```python
from build123d import *

# Parameters (mm, degrees)
F1_DEPTH = 120
F3_R     = 2
F4_R     = 3
F5_R     = 1.5


with BuildPart() as f1:
    # F0 (on Right) → F1 (new body)
    with BuildSketch(Plane.YZ):
        Polygon((-10, 19.4), (-10, 0), (0, 0), (0, 4), (-5.7, 4), (-5.7, 16.4), (-3.5, 16.4), (-3.5, 19.4), align=None)
    extrude(amount=F1_DEPTH)

    # F2: F1 across plane


with BuildPart() as f1_1:
    add(f1.part)
    add(f1.part.mirror(Plane.XZ))

    # F3
    f3_edges = [f1_1.edges().sort_by_distance(p)[0] for p in [
        (60, -5.7, 16.4),
        (60, -5.7, 4),
        (60, 5.7, 4),
        (60, 5.7, 16.4),
    ]]
    fillet(f3_edges, radius=F3_R)

    # F4
    f4_edges = [f1_1.edges().sort_by_distance(p)[0] for p in [
        (60, -10, 19.4),
        (60, 10, 19.4),
    ]]
    fillet(f4_edges, radius=F4_R)

    # F5
    f5_edges = [f1_1.edges().sort_by_distance(p)[0] for p in [
        (60, -3.5, 16.4),
        (60, 3.5, 16.4),
    ]]
    fillet(f5_edges, radius=F5_R)


solid = f1_1.part
```
Design review of the part built by this model. Coordinates are the model's own, in mm. A direction names the side the tool comes from. Coordinates: 2 decimals unless noted, no trailing zeros. Order: outer loops, then holes, each group sorted by start corner. A loop starts at its lowest first (then second) coordinate and runs counter-clockwise, first axis right, second up. Notation, with made-up numbers: (-24, 54.25) - (-9, 54.25) arc R27 cw to (-9, 92.25) - close; hole circle Ø9 at (-3, 29). An arc over 180 degrees is marked (long way). Answer in a Markdown table with one row per item.
(1) For faces 4 (the flat face through (59, 5.7, 10)), 5 (the flat face through (0, 0, 3)), list the 3-axis set-ups (+Z, -Z, +X, -X, +Y, -Y) from which the entire face can be reached by the end or side of a thin tool; tool diameter is ignored.
Checked values:
| item | result |
|---|---|
| face 4 | +X, -X |
| face 5 | +Z, -Z, -X, +Y, -Y |
(2) Consider section A-A on z = 7.5. State the section outline as (x, y) points.
Checked values:
| item | result |
|---|---|
| outline | (0, -10) - (120, -10) - (120, -5.7) - (0, -5.7) - close; (0, 5.7) - (120, 5.7) - (120, 10) - (0, 10) - close |
(3) Wall thickness on line 1 along Y through (x, z) = (101, 8.75); line 2 along Y through (x, z) = (61.5, 5.5); line 3 along Z through (x, y) = (88, 4): over which ranges is each line inside the solid? List them lowest first. Write a range as from..to.
Checked values:
| item | result |
|---|---|
| line 1 | -10..-5.7, 5.7..10 |
| line 2 | -10..-5.64, 5.64..10 |
| line 3 | 0..4.02, 16.53..19.4 |
(4) Clearance check with flat-ended pins moving along their axes: pin 1 (1.9 mm diameter, centred on x = 75, z = 18.5, fed in from -Y); pin 2 (0.5 mm diameter, centred on x = 64, z = 19, fed in from +Y). State where each tip first meets the part, or that it passes through.
Checked values:
| item | result |
|---|---|
| pin 1 | y = -9.77 |
| pin 2 | y = 8.86 |
(5) The part is to be moulded in two halves that separate along Z. For faces 1 (the flat face through (120, 0, 3)), 2 (the flat face through (59, 5, 19.4)), 3 (the cylindrical face through (60.84, -5.1, 4.57)), say which applies: released by +Z, released by -Z, zero draft, split by the parting line, or undercut.
Checked values:
| item | result |
|---|---|
| face 1 | zero draft |
| face 2 | released by +Z |
| face 3 | undercut |
(6) Consider section B-B on y = 0.5. State the section outline as (x, z) points, plus the area to 3 significant figures.
Checked values:
| item | result |
|---|---|
| outline | (0, 0) - (120, 0) - (120, 4) - (0, 4) - close |
| area | 480 mm^2 |
(7) Consider section C-C on y = -8.5. State the section outline as (x, z) points, plus the area to 3 significant figures.
Checked values:
| item | result |
|---|---|
| outline | (0, 0) - (120, 0) - (120, 19) - (0, 19) - close |
| area | 2,280 mm^2 |
